Check sheet for the modelled part. Datum: model origin and axes. Units: mm. A direction names the side the tool comes from. Coordinates: 2 decimals unless noted, no trailing zeros. Loops run counter-clockwise (first coordinate to the right, second up) from the corner with the lowest first, then second, coordinate; pieces in that order, holes last. Notation, with made-up numbers: (-27.5, 20) - (-23.5, 20) arc R17 ccw to (-23.5, 49) - close; hole circle Ø9 at (0, -5.75). An arc over 180 degrees is marked (long way). Answer as a JSON object with one key per item and string values. Group by question number.
Solid Edge part; units mm, degrees
sketch "Sketch1" plane through (0, 0, 0) normal (0, -1, 0) x (1, 0, 0)
  line L0 (-402.4784, 77.6999) -> (-342.4784, 77.6999)
  line L1 (-342.4784, 77.6999) -> (-342.4784, 677.6999)
  line L2 (-342.4784, 677.6999) -> (-402.4784, 677.6999)
  line L3 (-402.4784, 677.6999) -> (-402.4784, 77.6999)
  line L4 (-412.4784, 57.6999) -> (-332.4784, 57.6999)
  line L5 (-332.4784, 57.6999) -> (-332.4784, 787.6999)
  line L6 (-332.4784, 787.6999) -> (-412.4784, 787.6999)
  line L7 (-412.4784, 787.6999) -> (-412.4784, 57.6999)
  dimension "D1" = 402.4784
  dimension "D2" = 342.4784
  dimension "D3" = 332.4784
  dimension "D4" = 412.4784
extrude "Protrusion1" add sketch "Sketch1" against normal blind 50
sketch "Sketch2" plane through (-372.4784, 25, 77.6999) normal (0, 0, 1) x (1, 0, 0)
  circle A0 centre (0, 0) radius 10
extrude "Protrusion2" add sketch "Sketch2" along normal up to surface (600 mm away)
sketch "Sketch3" plane through (-372.4784, 50, 247.6999) normal (0, 1, 0) x (0, 0, 1)
  line L0 (490, -40) -> (540, -40)
  line L1 (540, -40) -> (540, 40)
  line L2 (540, 40) -> (490, 40)
  line L3 (490, 40) -> (490, -40)
  dimension "D1" = 490
  dimension "D2" = 540
extrude "ExtrudedProtrusion_3" add sketch "Sketch3" along normal blind 320
sketch "Sketch4" plane through (-372.4784, 310, 787.6999) normal (0, 0, 1) x (0, 1, 0)
  circle A0 centre (60, 0) radius 50
extrude "Cutout1" cut sketch "Sketch4" against normal through all
1. Release check for a two-part mould opening along X. For faces 5 (the face through (-372, 168, 787.7)), 6 (the face through (-412.478, 43, 533)), 7 (the face through (-372, 14, 677.7)) record: released by +X, released by -X, zero draft, split by the parting line, or undercut.
2. Gauge pin test, flat end, axial feed: pin 1 (12 mm diameter, centred on x = -381.5, z = 147, fed in from -Y). Record the tip position at first contact, or that the pin passes through.
3. Sectioned sample at A-A on y = 25. Record the cut outline in (x, z).
4. Material ranges on line 1 (Z direction, x = -350, y = 24.5); line 2 (X direction, y = 43, z = 665); line 3 (Z direction, x = -370, y = 198.5), recorded low to high.
5. Sectioned sample at D-D on x = -389.5. Record the cut outline in (y, z), plus the area to 3 significant figures.
6. Sectioned sample at B-B on z = 567.5. Record the cut outline in (x, y).
7. Access from +Z, -Z, +X, -X, +Y, -Y to the whole of each face (thin tool, end or side, straight path). Record for faces 1 (the face through (-372, 193, 737.7)), 2 (the face through (-373.127, 320.004, 763.05)), 3 (the face through (-402.478, 25, 382)), 4 (the face through (-373, 14, 77.7)).
8. Sectioned sample at C-C on x = -350.5. Record the cut outline in (y, z).
Answers follow:
{
 "1": {"face 5": "zero draft", "face 6": "released by -X", "face 7": "undercut"},
 "2": {"pin 1": "stops at y = 15.47"},
 "3": {"outline": "(-412.48, 57.7) - (-332.48, 57.7) - (-332.48, 787.7) - (-412.48, 787.7) - close; hole (-402.48, 77.7) - (-382.48, 77.7) - (-382.48, 677.7) - (-402.48, 677.7) - close; hole (-362.48, 77.7) - (-342.48, 77.7) - (-342.48, 677.7) - (-362.48, 677.7) - close"},
 "4": {"line 1": "z = 57.7 to 77.7, 677.7 to 787.7", "line 2": "x = -412.48 to -402.48, -342.48 to -332.48", "line 3": "z = 737.7 to 787.7"},
 "5": {"outline": "(0, 57.7) - (50, 57.7) - (50, 77.7) - (0, 77.7) - close; (0, 677.7) - (50, 677.7) - (50, 737.7) - (322.99, 737.7) - (322.99, 787.7) - (0, 787.7) - close", "area": "20,100 mm^2"},
 "6": {"outline": "(-412.48, 0) - (-402.48, 0) - (-402.48, 50) - (-412.48, 50) - close; circle Ø20 at (-372.48, 25); (-342.48, 0) - (-332.48, 0) - (-332.48, 50) - (-342.48, 50) - close"},
 "7": {"face 1": "-Z, +X, -X, +Y", "face 2": "+Z, -Z, +Y", "face 3": "+Y, -Y", "face 4": "none"},
 "8": {"outline": "(0, 57.7) - (50, 57.7) - (50, 77.7) - (0, 77.7) - close; (0, 677.7) - (50, 677.7) - (50, 737.7) - (325.09, 737.7) - (325.09, 787.7) - (0, 787.7) - close"}
}
